For this review, take the finished solid that the model builds, in its own axes (mm). A direction names the side the tool comes from. Coordinates: 2 decimals unless noted, no trailing zeros. Write each loop counter-clockwise with the first axis right and the second up, starting at its lowest first coordinate (ties: lowest second). Pieces come first, ordered by that corner, then holes.
```python
from build123d import *

# Parameters (mm, degrees)
CROQUIS1_R              = 5.25
SALIENTE_EXTRUIR1_DEPTH = 7.5


with BuildPart() as part:
    # Croquis1 → Saliente-Extruir1 (new body)
    with BuildSketch(Plane(origin=(0, 0, 0), x_dir=(1, 0, 0), z_dir=(0, 1, 0))):
        with BuildLine():
            Line((-2.5, 15), (-0.96403744, 18.894029408))
            Line((-0.96403744, 18.894029408), (0.96403744, 18.894029408))
            Line((0.96403744, 18.894029408), (2.5, 15))
            Line((2.5, 15), (2.588781311, 14.774918319))
            ThreePointArc((2.588781311, 14.774918319), (3.118675362, 14.672214011), (3.644531271, 14.550511737))
            Line((3.644531271, 14.550511737), (3.817186002, 14.720023472))
            Line((3.817186002, 14.720023472), (6.804202071, 17.652664095))
            Line((6.804202071, 17.652664095), (8.56558612, 16.86844539))
            Line((8.56558612, 16.86844539), (8.38491329, 12.686340257))
            Line((8.38491329, 12.686340257), (8.374470086, 12.444607297))
            ThreePointArc((8.374470086, 12.444607297), (8.816778784, 12.135254916), (9.247671287, 11.810189489))
            Line((9.247671287, 11.810189489), (9.474345866, 11.894821159))
            Line((9.474345866, 11.894821159), (13.39593323, 13.35899279))
            Line((13.39593323, 13.35899279), (14.686067144, 11.926153919))
            Line((14.686067144, 11.926153919), (12.819998898, 8.179097032))
            Line((12.819998898, 8.179097032), (12.712136904, 7.962510618))
            ThreePointArc((12.712136904, 7.962510618), (12.990381057, 7.5), (13.251804925, 7.027778186))
            Line((13.251804925, 7.027778186), (13.493305258, 7.012896206))
            Line((13.493305258, 7.012896206), (17.671385836, 6.755430269))
            Line((17.671385836, 6.755430269), (18.26719374, 4.92172209))
            Line((18.26719374, 4.92172209), (15.03839023, 2.257613625))
            Line((15.03839023, 2.257613625), (14.851759765, 2.103623516))
            ThreePointArc((14.851759765, 2.103623516), (14.917828431, 1.567926949), (14.964581102, 1.030200189))
            Line((14.964581102, 1.030200189), (15.179149589, 0.918377789))
            Line((15.179149589, 0.918377789), (18.891295291, -1.016207517))
            Line((18.891295291, -1.016207517), (18.689756586, -2.933720201))
            Line((18.689756586, -2.933720201), (14.656507272, -4.054231687))
            Line((14.656507272, -4.054231687), (14.423378438, -4.118999203))
            ThreePointArc((14.423378438, -4.118999203), (14.265847744, -4.635254916), (14.089845258, -5.145508779))
            Line((14.089845258, -5.145508779), (14.240381057, -5.334936491))
            Line((14.240381057, -5.334936491), (16.844728168, -8.612133791))
            Line((16.844728168, -8.612133791), (15.880690727, -10.281895618))
            Line((15.880690727, -10.281895618), (11.740381057, -9.665063509))
            Line((11.740381057, -9.665063509), (11.501063947, -9.629409539))
            ThreePointArc((11.501063947, -9.629409539), (11.147172382, -10.036959095), (10.778847167, -10.431512534))
            Line((10.778847167, -10.431512534), (10.83932127, -10.665791785))
            Line((10.83932127, -10.665791785), (11.885554515, -14.718943894))
            Line((11.885554515, -14.718943894), (10.32570917, -15.852237874))
            Line((10.32570917, -15.852237874), (6.794236298, -13.604718046))
            Line((6.794236298, -13.604718046), (6.590111016, -13.474807486))
            ThreePointArc((6.590111016, -13.474807486), (6.101049646, -13.703181865), (5.604088477, -13.913813005))
            Line((5.604088477, -13.913813005), (5.564044364, -14.152434784))
            Line((5.564044364, -14.152434784), (4.87126051, -18.28071488))
            Line((4.87126051, -18.28071488), (2.985318691, -18.681584188))
            Line((2.985318691, -18.681584188), (0.67330636, -15.191993238))
            Line((0.67330636, -15.191993238), (0.539668021, -14.990288804))
            ThreePointArc((0.539668021, -14.990288804), (0, -15), (-0.539668021, -14.990288804))
            Line((-0.539668021, -14.990288804), (-0.67330636, -15.191993238))
            Line((-0.67330636, -15.191993238), (-2.985318691, -18.681584188))
            Line((-2.985318691, -18.681584188), (-4.87126051, -18.28071488))
            Line((-4.87126051, -18.28071488), (-5.564044364, -14.152434784))
            Line((-5.564044364, -14.152434784), (-5.604088477, -13.913813005))
            ThreePointArc((-5.604088477, -13.913813005), (-6.101049646, -13.703181865), (-6.590111016, -13.474807486))
            Line((-6.590111016, -13.474807486), (-6.794236298, -13.604718046))
            Line((-6.794236298, -13.604718046), (-10.32570917, -15.852237874))
            Line((-10.32570917, -15.852237874), (-11.885554515, -14.718943894))
            Line((-11.885554515, -14.718943894), (-10.83932127, -10.665791785))
            Line((-10.83932127, -10.665791785), (-10.778847167, -10.431512534))
            ThreePointArc((-10.778847167, -10.431512534), (-11.147172382, -10.036959095), (-11.501063947, -9.629409539))
            Line((-11.501063947, -9.629409539), (-11.740381057, -9.665063509))
            Line((-11.740381057, -9.665063509), (-15.880690727, -10.281895618))
            Line((-15.880690727, -10.281895618), (-16.844728168, -8.612133791))
            Line((-16.844728168, -8.612133791), (-14.240381057, -5.334936491))
            Line((-14.240381057, -5.334936491), (-14.089845258, -5.145508779))
            ThreePointArc((-14.089845258, -5.145508779), (-14.265847744, -4.635254916), (-14.423378438, -4.118999203))
            Line((-14.423378438, -4.118999203), (-14.656507272, -4.054231687))
            Line((-14.656507272, -4.054231687), (-18.689756586, -2.933720201))
            Line((-18.689756586, -2.933720201), (-18.891295291, -1.016207517))
            Line((-18.891295291, -1.016207517), (-15.179149589, 0.918377789))
            Line((-15.179149589, 0.918377789), (-14.964581102, 1.030200189))
            ThreePointArc((-14.964581102, 1.030200189), (-14.917828431, 1.567926949), (-14.851759765, 2.103623516))
            Line((-14.851759765, 2.103623516), (-15.03839023, 2.257613625))
            Line((-15.03839023, 2.257613625), (-18.26719374, 4.92172209))
            Line((-18.26719374, 4.92172209), (-17.671385836, 6.755430269))
            Line((-17.671385836, 6.755430269), (-13.493305258, 7.012896206))
            Line((-13.493305258, 7.012896206), (-13.251804925, 7.027778186))
            ThreePointArc((-13.251804925, 7.027778186), (-12.990381057, 7.5), (-12.712136904, 7.962510618))
            Line((-12.712136904, 7.962510618), (-12.819998898, 8.179097032))
            Line((-12.819998898, 8.179097032), (-14.686067144, 11.926153919))
            Line((-14.686067144, 11.926153919), (-13.39593323, 13.35899279))
            Line((-13.39593323, 13.35899279), (-9.474345866, 11.894821159))
            Line((-9.474345866, 11.894821159), (-9.247671287, 11.810189489))
            ThreePointArc((-9.247671287, 11.810189489), (-8.816778784, 12.135254916), (-8.374470086, 12.444607297))
            Line((-8.374470086, 12.444607297), (-8.38491329, 12.686340257))
            Line((-8.38491329, 12.686340257), (-8.56558612, 16.86844539))
            Line((-8.56558612, 16.86844539), (-6.804202071, 17.652664095))
            Line((-6.804202071, 17.652664095), (-3.817186002, 14.720023472))
            Line((-3.817186002, 14.720023472), (-3.644531271, 14.550511737))
            ThreePointArc((-3.644531271, 14.550511737), (-3.118675362, 14.672214011), (-2.588781311, 14.774918319))
            Line((-2.588781311, 14.774918319), (-2.5, 15))
        make_face()
        with Locations(Location((0, 0, 0), (0, 0, 270))):
            Circle(CROQUIS1_R, mode=Mode.SUBTRACT)
    extrude(amount=SALIENTE_EXTRUIR1_DEPTH)


solid = part.part
```
1) Consider section B-B (z = 0.5). Give the boundary of the cut face in (x, y).
2) The part is to be moulded in two halves that separate along X. For faces 1 (the face through (-4, 7.5, -5)), 2 (the face through (9, 4, -12)), 3 (the face through (14.268, 3.698, 4.628)), 4 (the face through (0, 4, 15)), say which applies: pulls with the +X half, pulls with the -X half, needs draft (parallel to the pull), parting line crosses it, or undercut.
3) Consider section A-A (x = 0). Give the boundary of the cut face in (y, z).
4) Tool access review of faces 5 (the face through (12.987, 3.698, -7.507)), 6 (the face through (-14.264, 3.698, 4.642)), 7 (the face through (6.11, 3.7, 13.7)), 8 (the face through (3.94, 3.7, 18.48)), 9 (the face through (-7.697, 3.698, -17.255)): name each direction out of +Z, -Z, +X, -X, +Y, -Y from which nothing blocks a thin tool from reaching the whole face with its end or side.
5) Consider section C-C (z = -9). Give the boundary of the cut face in (x, y), then the cut area to 3 significant figures.
6) Clearance check with flat-ended pins moving along their axes: P1, Ø8.5, axis at x = 0, z = 0, coming from the +Y side; P2, Ø1, axis at y = 6.5, z = 0, coming from the +X side; P3, Ø4, axis at y = 3, z = 9, coming from the +X side. State where each tip first meets the part, or that it passes through.
7) For L1, parallel to X at y = 1.5, z = 14.5; L2, parallel to X at y = 0.75, z = -17; L3, parallel to Z at x = -3, y = 1, list the stretches that pass through material, from the lowest coordinate up.
Results:
1. outline: (-17.9, 0) - (-5.23, 0) - (-5.23, 7.5) - (-17.9, 7.5) - close; (5.23, 0) - (17.9, 0) - (17.9, 7.5) - (5.23, 7.5) - close
2. face 1: needs draft
2. face 2: undercut
2. face 3: pulls with the +X half
2. face 4: undercut
3. outline: (0, -18.89) - (7.5, -18.89) - (7.5, -5.25) - (0, -5.25) - close; (0, 5.25) - (7.5, 5.25) - (7.5, 15) - (0, 15) - close
4. face 5: +X, +Y, -Y
4. face 6: -X, +Y, -Y
4. face 7: +Z, +Y, -Y
4. face 8: +Z, +X, +Y, -Y
4. face 9: -Z, -X, +Y, -Y
5. outline: (-13.23, 0) - (13.23, 0) - (13.23, 7.5) - (-13.23, 7.5) - close
5. area: 198 mm2
6. P1: passes through
6. P2: stops at x = 17.9
6. P3: stops at x = 16.84
7. L1: x = -11.83 to -8.2, -5.51 to 5.51, 8.2 to 11.83
7. L2: x = -8.27 to -6.14, -1.71 to 1.71, 6.14 to 8.27
7. L3: z = -14.7 to -4.31, 4.31 to 18.68
